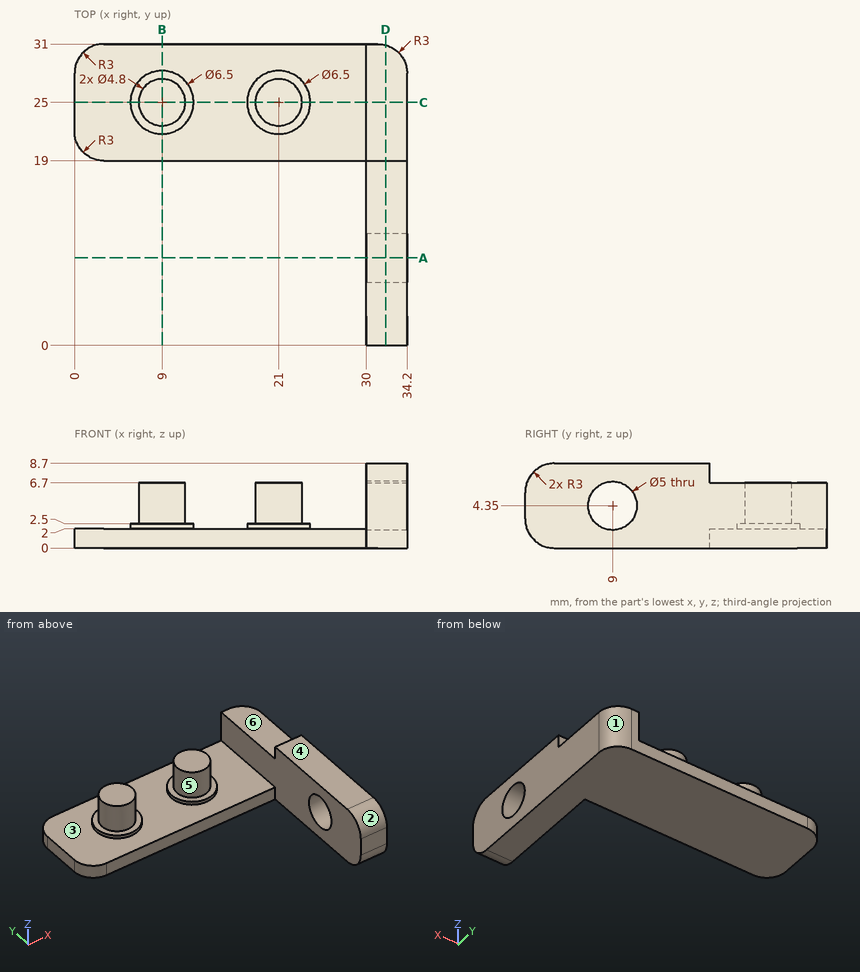
Design review of the part shown in the three views and the two pictorial views. Dimensions are in mm from the part's minimum x, y and z. A direction names the side the tool comes from. Round coordinates to 2 decimals unless told otherwise and drop trailing zeros. Write each loop counter-clockwise with the first axis right and the second up, starting at its lowest first coordinate (ties: lowest second). Pieces come first, ordered by that corner, then holes. Notation, with made-up numbers: (-37, -39.75) -> (-31, -39.75) arc R35 ccw to (-31, -0.75) -> close; hole circle Ø6 at (1, 2.25). An arc over 180 degrees is marked (long way). Write item = value, one per line. Start each with the question number.
1) Take a section at A-A, the plane y = 9. State the section outline as (x, z) points.
2) Take a section at D-D, the plane x = 32. State the section outline as (y, z) points, plus the area to 3 significant figures.
3) Take a section at B-B, the plane x = 9. State the section outline as (y, z) points, plus the area to 3 significant figures.
4) Tool access review of the marked faces 4, 5 and 6: name each direction out of +Z, -Z, +X, -X, +Y, -Y from which nothing blocks a thin tool from reaching the whole face with its end or side.
5) Clearance check with flat-ended pins moving along their axes: pin 1 (5 mm diameter, centred on x = 10, y = 23.5, fed in from +Z); pin 2 (1 mm diameter, centred on x = 32.5, z = 8, fed in from +Y); pin 3 (1.6 mm diameter, centred on x = 17.5, z = 0.5, fed in from -Y); pin 4 (1 mm diameter, centred on x = 28.5, y = 4.5, fed in from +Z). State where each tip first meets the part, or that it passes through.
6) Take a section at C-C, the plane y = 25. State the section outline as (x, z) points, plus the area to 3 significant figures.
7) Wall thickness on probe 1 along Z at (x, y) = (31, 9); probe 2 along Z at (x, y) = (14.5, 26); probe 3 along X at (y, z) = (22, 2.25): over which ranges is each line inside the solid? List them lowest first. Write a range as from..to.
8) Mouldability with a two-part tool opening along X and no side actions: class the marked faces 1, 2 and 3 as +X half, -X half, draft (parallel to the pull), parting line (faces both ways), or undercut.
Results list:
q1.outline = (30, 0) -> (34.2, 0) -> (34.2, 1.85) -> (30, 1.85) -> close; (30, 6.85) -> (34.2, 6.85) -> (34.2, 8.7) -> (30, 8.7) -> close
q2.outline = (0, 3) arc R3 ccw to (3, 0) -> (30.89, 0) -> (30.89, 6.7) -> (19, 6.7) -> (19, 8.7) -> (3, 8.7) arc R3 ccw to (0, 5.7) -> close; hole circle Ø5 at (9, 4.35)
q2.area = 221 mm²
q3.outline = (19, 0) -> (31, 0) -> (31, 2) -> (28.25, 2) -> (28.25, 2.5) -> (27.4, 2.5) -> (27.4, 6.7) -> (22.6, 6.7) -> (22.6, 2.5) -> (21.75, 2.5) -> (21.75, 2) -> (19, 2) -> close
q3.area = 47.4 mm²
q4.face_4 = +Z, +X, -X, +Y, -Y
q4.face_5 = +Z
q4.face_6 = +Z, +X, -X, +Y
q5.pin_1 = 6.7
q5.pin_2 = 19
q5.pin_3 = 19
q5.pin_4 = through
q6.outline = (0, 0) -> (34.2, 0) -> (34.2, 6.7) -> (30, 6.7) -> (30, 2) -> (24.25, 2) -> (24.25, 2.5) -> (23.4, 2.5) -> (23.4, 6.7) -> (18.6, 6.7) -> (18.6, 2.5) -> (17.75, 2.5) -> (17.75, 2) -> (12.25, 2) -> (12.25, 2.5) -> (11.4, 2.5) -> (11.4, 6.7) -> (6.6, 6.7) -> (6.6, 2.5) -> (5.75, 2.5) -> (5.75, 2) -> (0, 2) -> close
q6.area = 135 mm²
q7.probe_1 = 0..1.85, 6.85..8.7
q7.probe_2 = 0..2
q7.probe_3 = 7.75..10.25, 19.75..22.25, 30..34.2
q8.face_1 = +X half
q8.face_2 = draft
q8.face_3 = undercut
